Build history of the part. All positions in model axes, mm. Face numbers are marked on the shaded views. A direction names the side the tool comes from. Give positions to 0.01 mm unless a question says otherwise; leave off trailing zeros. Order: outer loops, then holes, each group sorted by start corner. A loop starts at its lowest first (then second) coordinate and runs counter-clockwise, first axis right, second up. Notation, with made-up numbers: (36, 60.25) - (67, 60.25) arc R19 cw to (67, 96.25) - close; hole circle Ø8 at (-18.75, 88). An arc over 180 degrees is marked (long way). Write each question's results on one line, items separated by ' | '. Start each with the question number.
1) Cut at B-B on x = -3. List the corners of the cut face in (y, z), plus the area to 3 significant figures.
2) Drop flat-ended pins along their axis: pin 1 Ø1 at (x, y) = (6, -19) entering from +Z; pin 2 Ø12 at (x, z) = (6, -9) entering from -Y; pin 3 Ø1.5 at (x, y) = (7, -5) entering from -Z. Give the stop position or say it passes through.
3) Cut at C-C on y = -22. List the corners of the cut face in (x, z) (1 decimal).
4) Cut at A-A on z = 0. List the corners of the cut face in (x, y), plus the area to 3 significant figures.
5) Tool access for the marked faces 1 and 2: list every direction of +Z, -Z, +X, -X, +Y, -Y with a clear straight run to the whole face (end or side of a thin tool).
6) Cut at D-D on y = -13.5. List the corners of the cut face in (x, z).
7) Drill centre lines: line 1 along Y through (x, z) = (-6.5, -10.25); line 2 along Z through (x, y) = (-0.75, -23.5); line 3 along X through (y, z) = (-3, -5.25). Where is each one in solid material? Low to high. Write a range as from..to.
from build123d import *

# Parameters (mm, degrees)
F0_R     = 12.7
F0_R_2   = 6.35
F0_R_3   = 4.7625
F1_DEPTH = 12.7
F2_DEPTH = 19.05
F3_DEPTH = 31.75


with BuildPart() as f1:
    # F0 (on Front) → F1 (new body)
    with BuildSketch(Plane.XZ):
        Circle(F0_R)
        Circle(F0_R_2, mode=Mode.SUBTRACT)
        with Locations((-1.478096, 0)):
            Circle(F0_R_3)
        Circle(F0_R_2)
        with Locations((-1.478096, 0)):
            Circle(F0_R_3, mode=Mode.SUBTRACT)
    extrude(amount=F1_DEPTH)

    # F0 (on Front) → F2 (join)
    with BuildSketch(Plane.XZ):
        with Locations((-1.478096, 0)):
            Circle(F0_R_3)
        Circle(F0_R_2)
        with Locations((-1.478096, 0)):
            Circle(F0_R_3, mode=Mode.SUBTRACT)
    extrude(amount=F2_DEPTH)

    # F0 (on Front) → F3 (join)
    with BuildSketch(Plane.XZ):
        with Locations((-1.478096, 0)):
            Circle(F0_R_3)
    extrude(amount=F3_DEPTH)


solid = f1.part
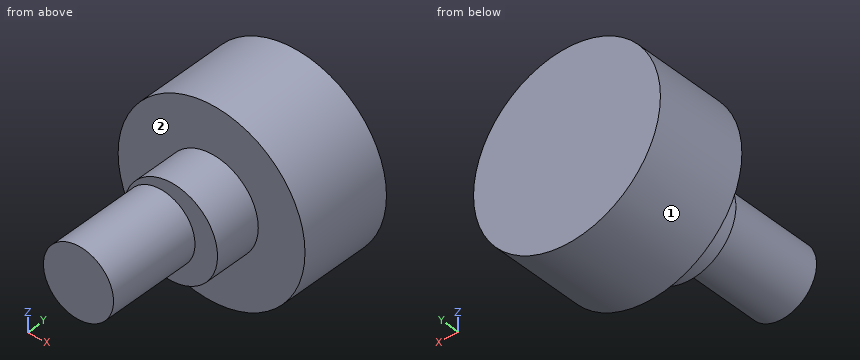
Results:
1) outline: (-31.75, -4.51) - (-19.05, -4.51) - (-19.05, -5.6) - (-12.7, -5.6) - (-12.7, -12.34) - (0, -12.34) - (0, 12.34) - (-12.7, 12.34) - (-12.7, 5.6) - (-19.05, 5.6) - (-19.05, 4.51) - (-31.75, 4.51) - close | area: 499 mm^2
2) pin 1: z = 3.17 | pin 2: y = -19.05 | pin 3: z = -11.06
3) outline: circle Ø9.5 at (-1.5, 0)
4) outline: (-12.7, -12.7) - (-6.35, -12.7) - (-6.35, -19.05) - (-6.24, -19.05) - (-6.24, -31.75) - (3.28, -31.75) - (3.28, -19.05) - (6.35, -19.05) - (6.35, -12.7) - (12.7, -12.7) - (12.7, 0) - (-12.7, 0) - close | area: 524 mm^2
5) face 1: +Y, -Y | face 2: -Y
6) outline: circle Ø12.7 at (0, 0)
7) line 1: -12.7..0 | line 2: -4.71..4.71 | line 3: -11.56..11.56
